from build123d import *

# Parameters (mm, degrees)
F0_W      = 100
F0_H      = 100
F1_DEPTH  = 45
F3_DEPTH  = 40
F5_DEPTH  = 85
F6_W      = 45
F6_H      = 20
F7_DEPTH  = 100.001
F9_DEPTH  = 100.001
F10_W     = 25
F10_H     = 30
F10_W_2   = 10
F11_DEPTH = 10


with BuildPart() as f1:
    # F0 (on Front) → F1 (new body)
    with BuildSketch(Plane.XZ):
        with Locations((-50, 50)):
            Rectangle(F0_W, F0_H)
    extrude(amount=F1_DEPTH)

    # F2 (on face) → F3 (cut)
    with BuildSketch(Plane.XY.offset(100)):
        Polygon((-100, -25), (-100, -45), (-65, -45), (-65, 0), (-85, 0), align=None)
    extrude(amount=-F3_DEPTH, mode=Mode.SUBTRACT)

    # F4 (on face) → F5 (cut)
    with BuildSketch(Plane.XY.offset(100)):
        Polygon((-50, 0), (-65, 0), (-65, -22.5), align=None)
    extrude(amount=-F5_DEPTH, mode=Mode.SUBTRACT)

    # F6 (on face) → F7 (cut, through all)
    with BuildSketch(Plane.XY.offset(100)):
        with Locations((-42.5, -35)):
            Rectangle(F6_W, F6_H)
    extrude(amount=-F7_DEPTH, mode=Mode.SUBTRACT)

    # F8 (on face) → F9 (cut, through all)
    with BuildSketch(Plane.XY.offset(100)):
        Polygon((0, 0), (-20, -25), (-20, -45), (0, -45), align=None)
    extrude(amount=-F9_DEPTH, mode=Mode.SUBTRACT)

    # F10 (on face) → F11 (cut)
    with BuildSketch(Plane.XZ.offset(25)):
        with Locations((-32.5, 45)):
            Rectangle(F10_W, F10_H)
        with Locations((-15, 45)):
            Rectangle(F10_W_2, F10_H)
    extrude(amount=-F11_DEPTH, mode=Mode.SUBTRACT)


solid = f1.part
Here's how the part is built. I have some questions about the finished solid (model axes, mm). A direction names the side the tool comes from. Round coordinates to 2 decimals unless told otherwise and drop trailing zeros. Order: outer loops, then holes, each group sorted by start corner. A loop starts at its lowest first (then second) coordinate and runs counter-clockwise, first axis right, second up. Notation, with made-up numbers: (31.25, 67) -> (43.25, 67) arc R16 ccw to (43.25, 78) -> close; hole circle Ø1 at (-4, 24.25). An arc over 180 degrees is marked (long way). Return JSON: item names as keys, results as strings.
Q1. If we section it at D-D on y = -19.5: List the corners of the cut face in (x, z) for me, plus the area to 3 significant figures.
Filled sheet:
{"outline": "(-100, 0) -> (-15.6, 0) -> (-15.6, 30) -> (-45, 30) -> (-45, 60) -> (-15.6, 60) -> (-15.6, 100) -> (-63, 100) -> (-63, 15) -> (-65, 15) -> (-65, 60) -> (-96.7, 60) -> (-96.7, 100) -> (-100, 100) -> close", "area": "6,120 mm^2"}
Q2. If we section it at C-C on z = 34: List the corners of the cut face in (x, y) for me, plus the area to 3 significant figures.
Filled sheet:
{"outline": "(-100, -45) -> (-65, -45) -> (-65, -25) -> (-45, -25) -> (-45, -15) -> (-12, -15) -> (0, 0) -> (-50, 0) -> (-65, -22.5) -> (-65, 0) -> (-100, 0) -> close", "area": "2,490 mm^2"}
Q3. If we section it at B-B on x = -18: List the corners of the cut face in (y, z) for me.
Filled sheet:
{"outline": "(-22.5, 0) -> (0, 0) -> (0, 100) -> (-22.5, 100) -> (-22.5, 60) -> (-15, 60) -> (-15, 30) -> (-22.5, 30) -> close"}
Q4. Which directions (+Z, -Z, +X, -X, +Y, -Y) give clear straight access to the entire face, cutting with the end or side of a thin tool? Please do faces 1 (the flat face through (-83, -22, 60)), 2 (the flat face through (-59, -9, 15)), 3 (the flat face through (-65, -24, 80)), 4 (the flat face through (-48, -25, 51)), 5 (the flat face through (-45, -20, 45)).
Filled sheet:
{"face 1": "+Z, -Y", "face 2": "+Z, +Y", "face 3": "+Z, +Y, -Y", "face 4": "+Z, -Z, +X, -Y", "face 5": "+X, -Y"}
Q5. If we section it at A-A on z = 93: List the corners of the cut face in (x, y) for me.
Filled sheet:
{"outline": "(-100, -25) -> (-85, 0) -> (-100, 0) -> close; (-65, -25) -> (-20, -25) -> (0, 0) -> (-50, 0) -> (-65, -22.5) -> close"}
Q6. For pin 1 Ø5 at (x, y) = (-23.5, -20) entering from -Z; pin 2 Ø18 at (y, z) = (-9.5, 38.5) entering from +X; pin 3 Ø8 at (x, z) = (-60, 46) entering from -Y; pin 4 Ø3 at (y, z) = (-30.5, 14) entering from +X, each with a flat end and sliding along its axis, tell me the tip position at first contact or that it passes through.
Filled sheet:
{"pin 1": "stops at z = 0", "pin 2": "stops at x = -0.4", "pin 3": "stops at y = -25", "pin 4": "stops at x = -65"}
Q7. If we mould it in two halves opening along Z, with no side actions, what happens to faces 6 (the flat face through (-65, -35, 30)), 7 (the flat face through (-32, -20, 30)), 8 (the flat face through (-33, -12, 100))? For each: released by +Z, released by -Z, zero draft, split by the parting line, or undercut.
Filled sheet:
{"face 6": "zero draft", "face 7": "undercut", "face 8": "released by +Z"}
Q8. I need wall thicknesses on line 1 along X through (y, z) = (-18.5, 51); line 2 along X through (y, z) = (-30.5, 6.5); line 3 along X through (y, z) = (-18, 64.5). Which ranges of each line are inside material? Lowest first, please. Write a range as from..to.
Filled sheet:
{"line 1": "x = -100..-65, -62.33..-45", "line 2": "x = -100..-65", "line 3": "x = -100..-95.8, -62..-14.4"}
